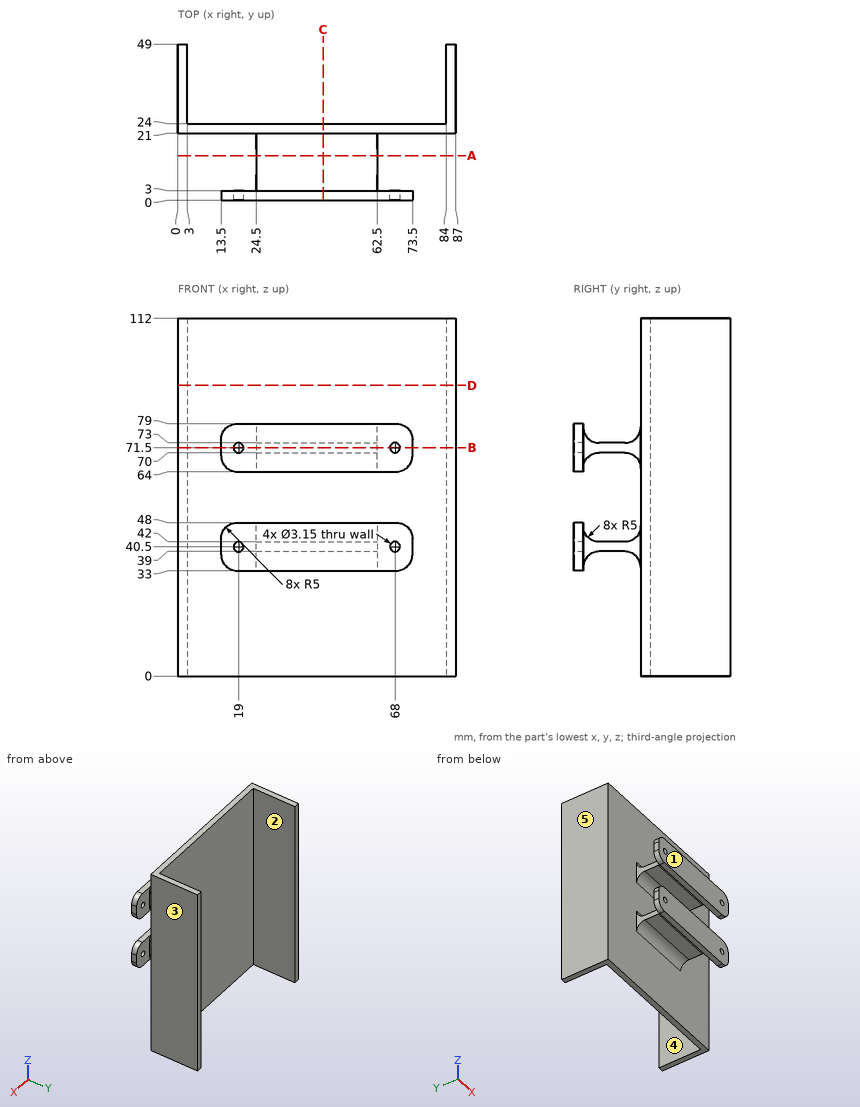
Geometry: see drawing. Coordinates: mm, zero at the bounding-box minimum. A direction names the side the tool comes from. Coordinates: 2 decimals unless noted, no trailing zeros. Write each loop counter-clockwise with the first axis right and the second up, starting at its lowest first coordinate (ties: lowest second). Pieces come first, ordered by that corner, then holes. Notation, with made-up numbers: M 66,59 L 100,59 A21 cw 100,79 Z; hole C -27.75,64 d5. An arc over 180 degrees is marked long. Answer as a JSON object with one key per item and string values.
1. Draft query along X for the marked faces 1, 2 and 3. Return one class per face: released by +X, released by -X, zero draft, split by the parting line, or undercut.
Evaluation:
{"face 1": "zero draft", "face 2": "undercut", "face 3": "released by +X"}
2. Cut plane B-B on z = 71.5. Output: boundary loops of the cut face in (x, y) (3 decimals).
Evaluation:
{"outline": "M 0,21 L 24.5,21 L 24.5,3 L 20.575,3 L 20.575,0 L 66.425,0 L 66.425,3 L 62.5,3 L 62.5,21 L 87,21 L 87,49 L 84,49 L 84,24 L 3,24 L 3,49 L 0,49 Z; M 13.5,0 L 17.425,0 L 17.425,3 L 13.5,3 Z; M 69.575,0 L 73.5,0 L 73.5,3 L 69.575,3 Z"}
3. Ray query, L1, parallel to X at y = 1.15, z = 40.5 (3 decimals); L2, parallel to Z at x = 68, y = 2 (3 decimals); L3, parallel to Z at x = 31, y = 19. Return the intervals inside material, ascending.
Evaluation:
{"L1": "13.5 to 17.425, 20.575 to 66.425, 69.575 to 73.5", "L2": "33 to 38.925, 42.075 to 48, 64 to 69.925, 73.075 to 79", "L3": "38 to 43, 69 to 74"}
4. Cut plane D-D on z = 91. Output: boundary loops of the cut face in (x, y), plus the area to 3 significant figures.
Evaluation:
{"outline": "M 0,21 L 87,21 L 87,49 L 84,49 L 84,24 L 3,24 L 3,49 L 0,49 Z", "area": "411 mm^2"}
5. Cut plane C-C on x = 45.5. Output: boundary loops of the cut face in (y, z), plus the area to 3 significant figures.
Evaluation:
{"outline": "M 0,33 L 3,33 L 3,34 A5 cw 8,39 L 16,39 A5 cw 21,34 L 21,0 L 24,0 L 24,112 L 21,112 L 21,78 A5 cw 16,73 L 8,73 A5 cw 3,78 L 3,79 L 0,79 L 0,64 L 3,64 L 3,65 A5 cw 8,70 L 16,70 A5 cw 21,65 L 21,47 A5 cw 16,42 L 8,42 A5 cw 3,47 L 3,48 L 0,48 Z", "area": "577 mm^2"}
6. Contact query for flat-ended pins moving along their axis: P1, Ø3.5, axis at x = 35.5, y = 1.5, coming from the -Z side; P2, Ø1.9, axis at x = 68, z = 40.5, coming from the -Y side; P3, Ø16.5, axis at x = 50.5, z = 40.5, coming from the +Y side. Output: stop coordinate, or through.
Evaluation:
{"P1": "z = 33", "P2": "y = 21", "P3": "y = 24"}
7. Access query for the marked faces 4 and 5. Directions: +Z, -Z, +X, -X, +Y, -Y. A direction counts if a zero-diameter tool reaches every point of the face in a straight line with its end or side. Return the directions, or none.
Evaluation:
{"face 4": "+Z, -Z, +Y", "face 5": "+Z, -Z, -X, +Y, -Y"}
8. Cut plane A-A on y = 14. Output: boundary loops of the cut face in (x, z), plus the area to 3 significant figures.
Evaluation:
{"outline": "M 24.5,39 L 62.5,39 L 62.5,42 L 24.5,42 Z; M 24.5,70 L 62.5,70 L 62.5,73 L 24.5,73 Z", "area": "228 mm^2"}
